from build123d import *

# Parameters (mm, degrees)
CYLINDER006_R     = 1.95
CYLINDER006_DEPTH = 6.2
POCKET_DEPTH      = 3.2
CHAMFER001_SIZE   = 0.1
CHAMFER002_SIZE   = 0.1


with BuildPart() as part:
    # Cylinder006 → Cylinder006 (new body)
    with BuildSketch(Plane.XY):
        Circle(CYLINDER006_R)
    extrude(amount=CYLINDER006_DEPTH)

    # Sketch001 (on Face2 of Cylinder006) → Pocket (cut)
    with BuildSketch(Plane.XY.offset(6.2)):
        Polygon((-1.1, -0.635085), (-1.1, 0.635085), (0, 1.270171), (1.1, 0.635085), (1.1, -0.635085), (0, -1.270171), align=None)
    extrude(amount=-POCKET_DEPTH, mode=Mode.SUBTRACT)

    # Chamfer001
    chamfer001_edges = [part.edges().sort_by_distance(p)[0] for p in [
        (-1.95, 0, 0),
    ]]
    chamfer(chamfer001_edges, length=CHAMFER001_SIZE)

    # Chamfer002
    chamfer002_edges = [part.edges().sort_by_distance(p)[0] for p in [
        (-1.95, 0, 6.2),
    ]]
    chamfer(chamfer002_edges, length=CHAMFER002_SIZE)


solid = part.part
Read the model definition and answer for the solid it produces. Units are mm, in the model's axes. A direction names the side the tool comes from. Round coordinates to 2 decimals unless told otherwise and drop trailing zeros. Loops run counter-clockwise (first coordinate to the right, second up) from the corner with the lowest first, then second, coordinate; pieces in that order, holes last.
Q1. Section B-B on y = 0 is taken. Write down the section's boundary in (x, z).
Q2. Consider probe 1 along Z at (x, y) = (-0.1, -0.1); probe 2 along X at (y, z) = (-0.5, 3.5); probe 3 along X at (y, z) = (-1.05, 5). Determine where each line is inside the solid, lowest interval first.
Q3. Which of the six approach directions +Z, -Z, +X, -X, +Y, -Y give full straight-line access (tool end or side, diameter ignored) to faces 4 (the face through (-1.1, 0, 5)), 5 (the face through (1, 1, 6.2))?
Q4. Section A-A on z = 3.75 is taken. Write down the section's boundary in (x, y).
Q5. Section C-C on z = 1.5 is taken. Write down the section's boundary in (x, y).
Q6. Each of these flat-tipped pins is pushed along its axis until it touches: pin 1 (1 mm diameter, centred on x = 0.5, z = 1.5, fed in from +Y); pin 2 (1.5 mm diameter, centred on y = -1, z = 2, fed in from +X). Where does it stop, or does it pass through?
Q7. Determine the mould class of faces 1 (the face through (-0.54, -0.96, 4.62)), 2 (the face through (-1.437, 1.318, 3.058)), 3 (the face through (0, 0, 0)) for opening direction Y: released by +Y, released by -Y, zero draft, split by the parting line, or undercut.
Output:
1. outline: (-1.95, 0.1) - (-1.85, 0) - (1.85, 0) - (1.95, 0.1) - (1.95, 6.1) - (1.85, 6.2) - (1.1, 6.2) - (1.1, 3) - (-1.1, 3) - (-1.1, 6.2) - (-1.85, 6.2) - (-1.95, 6.1) - close
2. probe 1: z = 0 to 3
2. probe 2: x = -1.88 to -1.1, 1.1 to 1.88
2. probe 3: x = -1.64 to -0.38, 0.38 to 1.64
3. face 4: +Z
3. face 5: +Z, +X, -X, +Y, -Y
4. outline: circle Ø3.9 at (0, 0); hole (-1.1, -0.64) - (0, -1.27) - (1.1, -0.64) - (1.1, 0.64) - (0, 1.27) - (-1.1, 0.64) - close
5. outline: circle Ø3.9 at (0, 0)
6. pin 1: stops at y = 1.95
6. pin 2: stops at x = 1.93
7. face 1: undercut
7. face 2: split by the parting line
7. face 3: zero draft
